Geometry: final body of the model. Coordinates: model frame, mm. A direction names the side the tool comes from. Round coordinates to 2 decimals unless told otherwise and drop trailing zeros. Order: outer loops, then holes, each group sorted by start corner. A loop starts at its lowest first (then second) coordinate and runs counter-clockwise, first axis right, second up. Notation, with made-up numbers: M 9,5 L 14,5 A13 ccw 14,16 Z; hole C -5,55 d11. An arc over 180 degrees is marked long. Put each result on its own line as item: value. Start each with the question number.
1) Material intervals for probe 1 along Y at (x, z) = (7.5, 1.4) (3 decimals); probe 2 along X at (y, z) = (-7, 1); probe 3 along Y at (x, z) = (-2.75, 24), sorted ascending. Write a range as [from, to].
2) Section D-D, the plane x = -6. Return loops of the section in (y, z), then the cut area to 3 significant figures.
3) Draft query along Y for faces 1 (the cylindrical face through (7.061, 5.523, 1.014)), 2 (the flat face through (0, 16, 45)), 3 (the cylindrical face through (-11.6, -14.14, 1.01)). Return one class per face: pulls with the +Y half, pulls with the -Y half, needs draft (parallel to the pull), parting line crosses it, or undercut.
4) First-contact query: P1, Ø4, axis at x = 9.5, z = 11, coming from the -Y side; P2, Ø2, axis at x = -6.5, y = -9, coming from the +Z side. Flat tips, straight axial feed; report the tip coordinate or a pass-through.
5) Section A-A, the plane x = 0. Return loops of the section in (y, z) (3 decimals).
6) Access query for faces 4 (the flat face through (0, 15, 24)), 5 (the cylindrical face through (-7.939, 5.523, 1.014)). Directions: +Z, -Z, +X, -X, +Y, -Y. A direction counts if a zero-diameter tool reaches every point of the face in a straight line with its end or side. Return the directions, or none.
7) Section B-B, the plane z = 33. Return loops of the section in (x, y) (3 decimals).
8) Section C-C, the plane y = -7.5. Return loops of the section in (x, z) (3 decimals).
from build123d import *

# Parameters (mm, degrees)
SKETCH1_W           = 25
SKETCH1_H           = 30
BOSS_EXTRUDE1_DEPTH = 2
SKETCH2_R           = 2.025
CUT_EXTRUDE1_DEPTH  = 20.627786426
SKETCH3_W           = 25
SKETCH3_H           = 2
BOSS_EXTRUDE2_DEPTH = 45
FILLET1_R           = 2
FILLET2_R           = 1
SKETCH4_R           = 7.025
CUT_EXTRUDE2_DEPTH  = 57.61492736
FILLET6_R           = 10
FILLET7_R           = 3


with BuildPart() as part:
    # Sketch1 → Boss-Extrude1 (new body)
    with BuildSketch(Plane.XY):
        Rectangle(SKETCH1_W, SKETCH1_H)
    extrude(amount=BOSS_EXTRUDE1_DEPTH)

    # Sketch2 → Cut-Extrude1 (cut, through all)
    with BuildSketch(Plane.XY.offset(2)):
        with Locations((-7.5, 7.5)):
            Circle(SKETCH2_R)
        with Locations((7.5, 7.5)):
            Circle(SKETCH2_R)
        with Locations((7.5, -7.5)):
            Circle(SKETCH2_R)
        with Locations((-7.5, -7.5)):
            Circle(SKETCH2_R)
    extrude(amount=-CUT_EXTRUDE1_DEPTH, mode=Mode.SUBTRACT)

    # Sketch3 → Boss-Extrude2 (add)
    with BuildSketch(Plane(origin=(0, 0, 0), x_dir=(-1, 0, 0), z_dir=(0, 0, -1))):
        with Locations((0, 16)):
            Rectangle(SKETCH3_W, SKETCH3_H)
    extrude(amount=-BOSS_EXTRUDE2_DEPTH)

    # Fillet1
    fillet1_edges = [part.edges().sort_by_distance(p)[0] for p in [
        (0, 17, 0),
    ]]
    fillet(fillet1_edges, radius=FILLET1_R)

    # Fillet2
    fillet2_edges = [part.edges().sort_by_distance(p)[0] for p in [
        (0, 15, 2),
    ]]
    fillet(fillet2_edges, radius=FILLET2_R)

    # Sketch4 → Cut-Extrude2 (cut, through all)
    with BuildSketch(Plane(origin=(0, 17, 0), x_dir=(1, 0, 0), z_dir=(0, 1, 0))):
        with Locations(Location((0, -33, 0), (0, 0, 270))):
            Circle(SKETCH4_R)
    extrude(amount=-CUT_EXTRUDE2_DEPTH, mode=Mode.SUBTRACT)

    # Fillet6
    fillet6_edges = [part.edges().sort_by_distance(p)[0] for p in [
        (12.5, 16, 45),
        (-12.5, 16, 45),
    ]]
    fillet(fillet6_edges, radius=FILLET6_R)

    # Fillet7
    fillet7_edges = [part.edges().sort_by_distance(p)[0] for p in [
        (12.5, -15, 1),
        (-12.5, -15, 1),
    ]]
    fillet(fillet7_edges, radius=FILLET7_R)


solid = part.part
Result sheet:
1. probe 1: y = [-15, -9.525], [-5.475, 5.475], [9.525, 16.908]
1. probe 2: x = [-12.5, -9.46], [-5.54, 5.54], [9.46, 12.5]
1. probe 3: y = [15, 17]
2. outline: M -15,0 L -8.86,0 L -8.86,2 L -15,2 Z; M -6.14,0 L 6.14,0 L 6.14,2 L -6.14,2 Z; M 8.86,0 L 15,0 A2 ccw 17,2 L 17,29.35 L 15,29.35 L 15,3 A1 cw 14,2 L 8.86,2 Z; M 15,36.65 L 17,36.65 L 17,44.37 L 15,44.37 Z
2. area: 123 mm2
3. face 1: undercut
3. face 2: needs draft
3. face 3: pulls with the -Y half
4. P1: stops at y = 15
4. P2: stops at z = 2
5. outline: M -15,0 L 15,0 A2 ccw 17,2 L 17,25.975 L 15,25.975 L 15,3 A1 cw 14,2 L -15,2 Z; M 15,40.025 L 17,40.025 L 17,45 L 15,45 Z
6. face 4: +Z, +X, -X, -Y
6. face 5: +Z, -Z
7. outline: M -12.5,15 L -7.025,15 L -7.025,17 L -12.5,17 Z; M 7.025,15 L 12.5,15 L 12.5,17 L 7.025,17 Z
8. outline: M -12.5,0 L -9.525,0 L -9.525,2 L -12.5,2 Z; M -5.475,0 L 5.475,0 L 5.475,2 L -5.475,2 Z; M 9.525,0 L 12.5,0 L 12.5,2 L 9.525,2 Z
